Geometry check sheet. Reference: drawing and pictorial views, mm from the part's lowest x, y, z. A direction names the side the tool comes from. Give positions to 0.01 mm unless a question says otherwise; leave off trailing zeros. Order: outer loops, then holes, each group sorted by start corner. A loop starts at its lowest first (then second) coordinate and runs counter-clockwise, first axis right, second up. Notation, with made-up numbers: (67.25, -31) -> (112.25, -31) arc R29 ccw to (112.25, 7) -> close; hole circle Ø3 at (11.5, 49.5). An arc over 180 degrees is marked (long way). Write each question's results on one line, items separated by ' | '. Start each with the question number.
1. Cross-section at C-C, the plane y = 28.75. Enter the section's corners in (x, z), then the cut area to 3 significant figures.
2. Mould release check, pull along Y, two halves, no side actions. Record for the marked faces 6, 7, 8 and 9: +Y half, -Y half, draft (parallel to the pull), parting line (faces both ways), or undercut.
3. Set-up check for the marked faces 1, 2, 3, 4 and 5: record each of +Z, -Z, +X, -X, +Y, -Y from which the full face is reachable in a straight line by a thin tool's end or side.
4. Cross-section at B-B, the plane z = 2. Enter the section's corners in (x, y), then the cut area to 3 significant figures.
5. Material ranges on L1, parallel to Y at x = 21, z = 1.75; L2, parallel to X at y = 28.75, z = 1.6; L3, parallel to Y at x = 1.5, z = 0.2, recorded low to high. Write a range as from..to.
6. Depth check by flat-ended pin: pin 1 Ø1.5 at (y, z) = (2, 1.5) entering from -X; pin 2 Ø0.9 at (x, z) = (1.5, 1) entering from +Y; pin 3 Ø1.5 at (x, z) = (3, 2) entering from -Y. Enter the tip coordinate at first touch or a pass-through.
7. Cross-section at D-D, the plane x = 21. Enter the section's corners in (y, z), then the cut area to 3 significant figures.
8. Cross-section at A-A, the plane x = 12.5. Enter the section's corners in (y, z), then the cut area to 3 significant figures.
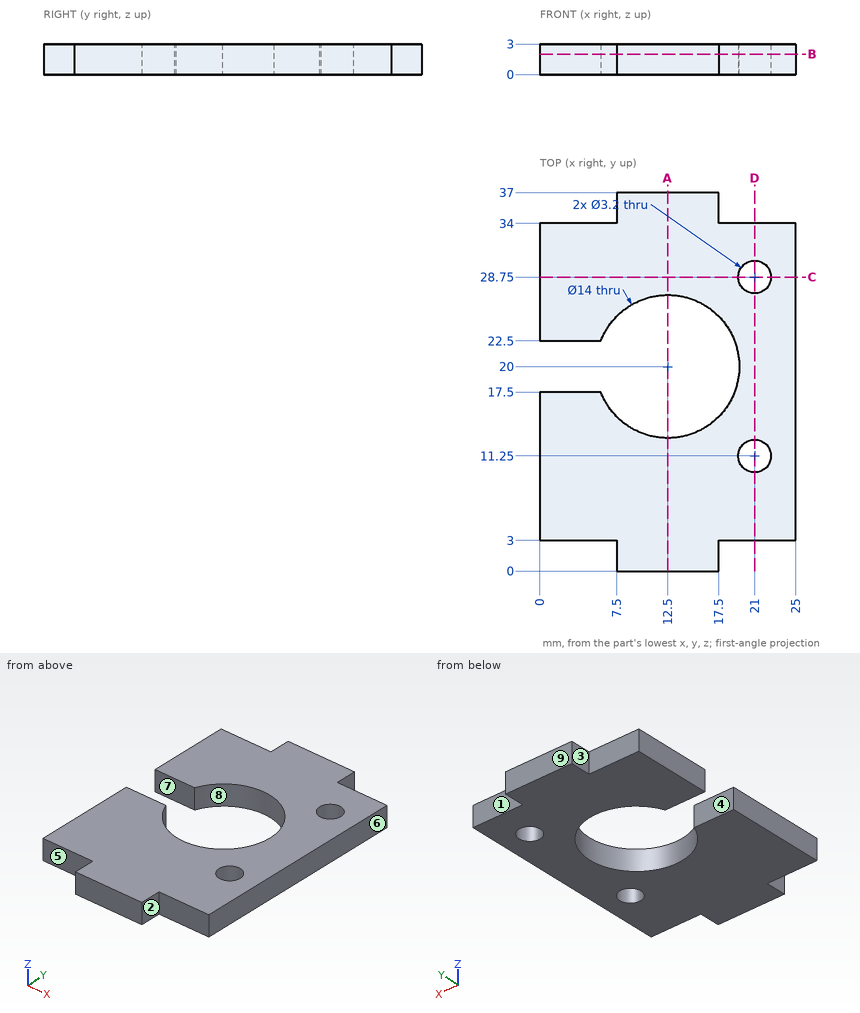
Results below:
1) outline: (0, 0) -> (19.4, 0) -> (19.4, 3) -> (0, 3) -> close; (22.6, 0) -> (25, 0) -> (25, 3) -> (22.6, 3) -> close | area: 65.4 mm²
2) face 6: draft | face 7: undercut | face 8: undercut | face 9: +Y half
3) face 1: +Z, -Z, +X, +Y | face 2: +Z, -Z, +X, -Y | face 3: +Z, -Z, -X, +Y | face 4: +Z, -Z, -X | face 5: +Z, -Z, -X, -Y
4) outline: (0, 3) -> (7.5, 3) -> (7.5, 0) -> (17.5, 0) -> (17.5, 3) -> (25, 3) -> (25, 34) -> (17.5, 34) -> (17.5, 37) -> (7.5, 37) -> (7.5, 34) -> (0, 34) -> (0, 22.5) -> (5.96, 22.5) arc R7 cw (long way) to (5.96, 17.5) -> (0, 17.5) -> close; hole circle Ø3.2 at (21, 11.25); hole circle Ø3.2 at (21, 28.75) | area: 637 mm²
5) L1: y = 3..9.65, 12.85..27.15, 30.35..34 | L2: x = 0..19.4, 22.6..25 | L3: y = 3..17.5, 22.5..34
6) pin 1: stops at x = 7.5 | pin 2: stops at y = 34 | pin 3: stops at y = 3
7) outline: (3, 0) -> (9.65, 0) -> (9.65, 3) -> (3, 3) -> close; (12.85, 0) -> (27.15, 0) -> (27.15, 3) -> (12.85, 3) -> close; (30.35, 0) -> (34, 0) -> (34, 3) -> (30.35, 3) -> close | area: 73.8 mm²
8) outline: (0, 0) -> (13, 0) -> (13, 3) -> (0, 3) -> close; (27, 0) -> (37, 0) -> (37, 3) -> (27, 3) -> close | area: 69.0 mm²
